Source: CAD feature listing. Evaluate the final solid. Frame: model axes, mm. A direction names the side the tool comes from. Give positions to 0.01 mm unless a question says otherwise; leave off trailing zeros. Write each loop counter-clockwise with the first axis right and the second up, starting at its lowest first coordinate (ties: lowest second). Pieces come first, ordered by that corner, then holes. Notation, with made-up numbers: M -29.75,3 L 14.25,3 A25 cw 14.25,23 Z; hole C 28.5,10 d4. An arc over 180 degrees is marked long. Use CSV: the item, a comma, the result in double quotes. Start each with the question number.
from build123d import *

# Parameters (mm, degrees)
F0_W           = 105
F0_H           = 15
F1_DEPTH       = 5
F2_W           = 103
F2_H           = 13
F3_DEPTH       = 15
F5_D           = 4.2
F5_DEPTH       = 8
F5_TIP         = 1.2618073
F7_D           = 5.5
F7_CBORE_D     = 9.5
F7_CBORE_DEPTH = 5.4
F8_SIZE        = 1


with BuildPart() as f1:
    # F0 (on Top) → F1 (new body)
    with BuildSketch(Plane.XY):
        with Locations((52.5, 7.5)):
            Rectangle(F0_W, F0_H)
    extrude(amount=F1_DEPTH)

    # F2 (on face) → F3 (join)
    with BuildSketch(Plane.XY.offset(5)):
        with Locations((53.5, 8.5)):
            Rectangle(F2_W, F2_H)
    extrude(amount=F3_DEPTH)

    # F5
    with Locations(Plane.YZ.offset(105)):
        with Locations((7.5, 10)):
            Hole(F5_D / 2, depth=F5_DEPTH)
            with Locations((0, 0, -(F5_DEPTH + F5_TIP / 2))):  # 118° drill point
                Cone(0, F5_D / 2, F5_TIP, mode=Mode.SUBTRACT)

    # F7 (through all)
    with Locations(Plane.XZ.offset(-2)):
        with Locations((10, 10)):
            CounterBoreHole(F7_D / 2, F7_CBORE_D / 2, F7_CBORE_DEPTH)

    # F8
    f8_edges = [f1.edges().sort_by_distance(p)[0] for p in [
        (53.5, 2, 20),
        (53.5, 15, 20),
        (105, 8.5, 20),
        (2, 8.5, 20),
    ]]
    chamfer(f8_edges, length=F8_SIZE)


solid = f1.part
Item 1: Pull-direction query (Z, two-part tool) for faces 1 (the flat face through (13, 7.4, 10)), 2 (the flat face through (53, 9, 20)), 3 (the flat face through (105, 7, 7)); classes: released by +Z, released by -Z, zero draft, split by the parting line, or undercut.
Item 2: Section A-A (x = 10). Return the cut outline in (y, z).
Item 3: Section C-C (x = 48.5). Return the cut outline in (y, z), plus the area to 3 significant figures.
Item 4: Section B-B (y = 12). Return the cut outline in (x, z), plus the area to 3 significant figures.
Item 5: Material intervals for probe 1 along Z at (x, y) = (10, 5.4); probe 2 along Z at (x, y) = (10, 9.5); probe 3 along Y at (x, z) = (61, 11.5), sorted ascending.
Item 6: Contact query for flat-ended pins moving along their axis: pin 1 Ø8.5 at (x, z) = (10, 10) entering from -Y; pin 2 Ø5 at (x, z) = (10, 10) entering from +Y; pin 3 Ø4 at (x, z) = (72.5, 13) entering from -Y; pin 4 Ø1 at (y, z) = (11, 16.5) entering from -X. Output: stop coordinate, or through.
Item 7: Set-up query: faces 4 (the flat face through (2, 8, 12)), 5 (the cylindrical face through (100.944, 7.773, 12.082)), 6 (the flat face through (53, 2, 12)), 7 (the cylindrical face through (8.97, 4.662, 5.363)), 8 (the flat face through (44, 1, 5)). Return all of +Z, -Z, +X, -X, +Y, -Y with unobstructed straight access to the full face (end or side cutting, diameter ignored); none if empty.
Item 8: Section D-D (y = 4). Return the cut outline in (x, z), plus the area to 3 significant figures.
Output values:
1,face 1,"undercut"
1,face 2,"released by +Z"
1,face 3,"zero draft"
2,outline,"M 0,0 L 15,0 L 15,7.25 L 7.4,7.25 L 7.4,5.25 L 2,5.25 L 2,5 L 0,5 Z; M 2,14.75 L 7.4,14.75 L 7.4,12.75 L 15,12.75 L 15,19 L 14,20 L 3,20 L 2,19 Z"
3,outline,"M 0,0 L 15,0 L 15,19 L 14,20 L 3,20 L 2,19 L 2,5 L 0,5 Z"
3,area,"269 mm2"
4,outline,"M 0,0 L 105,0 L 105,19 L 104,20 L 3,20 L 2,19 L 2,5 L 0,5 Z; hole C 10,10 d5.5"
4,area,"2,050 mm2"
5,probe 1,"z = 0 to 5.25, 14.75 to 20"
5,probe 2,"z = 0 to 7.25, 12.75 to 20"
5,probe 3,"y = 2 to 15"
6,pin 1,"stops at y = 7.4"
6,pin 2,"passes through"
6,pin 3,"stops at y = 2"
6,pin 4,"stops at x = 2"
7,face 4,"+Z, -X, +Y, -Y"
7,face 5,"+X"
7,face 6,"+Z, +X, -X, -Y"
7,face 7,"-Y"
7,face 8,"+Z, -X, -Y"
8,outline,"M 0,0 L 105,0 L 105,19 L 104,20 L 3,20 L 2,19 L 2,5 L 0,5 Z; hole C 10,10 d9.5"
8,area,"2,000 mm2"
